Read the model definition and answer for the solid it produces. Units are mm, in the model's axes. Face numbers are marked on the shaded views. A direction names the side the tool comes from. Coordinates: 2 decimals unless noted, no trailing zeros. Write each loop counter-clockwise with the first axis right and the second up, starting at its lowest first coordinate (ties: lowest second). Pieces come first, ordered by that corner, then holes.
(1) Section D-D on y = -5.5 is taken. Write down the section's boundary in (x, z).
(2) Section A-A on y = -57.57 is taken. Write down the section's boundary in (x, z).
(3) The mould has two halves that part along X. Classify the marked faces 4, 5 and 6: +X half, -X half, draft (parallel to the pull), parting line (faces both ways), or undercut.
(4) Section B-B on x = -39.82 is taken. Write down the section's boundary in (y, z).
(5) Given pin 1 (11.5 mm diameter, centred on x = -6, y = -57.57, fed in from +Z); pin 2 (5.5 mm diameter, centred on y = -33, z = -476, fed in from -X); pin 3 (9.5 mm diameter, centred on x = -6, y = -36, fed in from -Z), each flat-ended and moving along its own axis, determine where each tip first touches the part or whether it passes through.
(6) Which of the six approach directions +Z, -Z, +X, -X, +Y, -Y give full straight-line access (tool end or side, diameter ignored) to the marked faces 1, 2 and 3?
(7) Find the intervals of material crossed by probe 1 along Y at (x, z) = (-15, -477.25); probe 2 along X at (y, z) = (-26, -478); probe 3 along Y at (x, z) = (-6.5, -477), in increasing order.
(8) Section C-C on z = -479 is taken. Write down the section's boundary in (x, y), then the cut area to 3 significant figures.
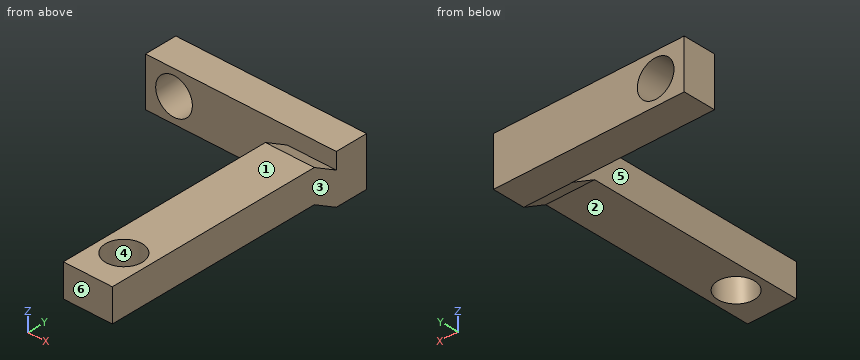
from build123d import *

# Parameters (mm, degrees)
BOSS_EXTRUDE1_DEPTH = 12
BOSS_EXTRUDE2_DEPTH = 46.82
SKETCH3_R           = 4.5
CUT_EXTRUDE2_DEPTH  = 8
SKETCH5_R           = 4.5
CUT_EXTRUDE4_DEPTH  = 8


with BuildPart() as part:
    # Sketch1 → Boss-Extrude1 (new body)
    with BuildSketch(Plane(origin=(0, 0, 0), x_dir=(0, 0, -1), z_dir=(1, 0, 0))):
        Polygon((475.915980223, -8), (483.915980223, -8), (480.565980223, -13.802370205), (480.565980223, -67.07), (472.565980223, -67.07), (472.565980223, -13.802370205), align=None)
    extrude(amount=-BOSS_EXTRUDE1_DEPTH)

    # Sketch1<3> → Boss-Extrude2 (add)
    with BuildSketch(Plane(origin=(0, 0, 0), x_dir=(0, 0, -1), z_dir=(1, 0, 0))):
        Polygon((471.915980223, -8), (475.915980223, -8), (483.915980223, -8), (483.915980223, 0), (471.915980223, 0), align=None)
    extrude(amount=-BOSS_EXTRUDE2_DEPTH)

    # Sketch3 → Cut-Extrude2 (cut)
    with BuildSketch(Plane.XZ.offset(8)):
        with Locations(Location((-39.82, -477.915980223, 0), (0, 0, 270))):
            Circle(SKETCH3_R)
    extrude(amount=-CUT_EXTRUDE2_DEPTH, mode=Mode.SUBTRACT)

    # Sketch5 → Cut-Extrude4 (cut)
    with BuildSketch(Plane.XY.offset(-472.565980223)):
        with Locations((-6, -57.57)):
            Circle(SKETCH5_R)
    extrude(amount=-CUT_EXTRUDE4_DEPTH, mode=Mode.SUBTRACT)


solid = part.part
Response:
1. outline: (-46.82, -483.92) - (0, -483.92) - (0, -471.92) - (-46.82, -471.92) - close; hole circle Ø9 at (-39.82, -477.92)
2. outline: (-12, -480.57) - (-10.5, -480.57) - (-10.5, -472.57) - (-12, -472.57) - close; (-1.5, -480.57) - (0, -480.57) - (0, -472.57) - (-1.5, -472.57) - close
3. face 4: undercut
3. face 5: -X half
3. face 6: draft
4. outline: (-8, -483.92) - (0, -483.92) - (0, -482.42) - (-8, -482.42) - close; (-8, -473.42) - (0, -473.42) - (0, -471.92) - (-8, -471.92) - close
5. pin 1: stops at z = -472.57
5. pin 2: stops at x = -12
5. pin 3: stops at z = -480.57
6. face 1: +Z, +X, -X, -Y
6. face 2: -Z, +X, -X, -Y
6. face 3: +Z, -Z, +X, +Y, -Y
7. probe 1: y = -8 to 0
7. probe 2: x = -12 to 0
7. probe 3: y = -67.07 to -62.04, -53.1 to 0
8. outline: (-46.82, -8) - (-44.19, -8) - (-44.19, 0) - (-46.82, 0) - close; (-35.45, -8) - (-12, -8) - (-12, -67.07) - (0, -67.07) - (0, 0) - (-35.45, 0) - close; hole circle Ø9 at (-6, -57.57)
8. area: 950 mm2
